Geometry check sheet. Reference: the model listing, model coordinates, mm. Face numbers are marked on the shaded views. A direction names the side the tool comes from. Coordinates: 2 decimals unless noted, no trailing zeros. Loops run counter-clockwise (first coordinate to the right, second up) from the corner with the lowest first, then second, coordinate; pieces in that order, holes last.
from build123d import *

# Parameters (mm, degrees)
SKETCH2_W           = 112.2
SKETCH2_H           = 87.2
SKETCH2_R           = 3
SKETCH2_W_2         = 71
SKETCH2_H_2         = 24
BOSS_EXTRUDE2_DEPTH = 60
SKETCH6_W           = 105
SKETCH6_H           = 80
CUT_EXTRUDE4_DEPTH  = 57.6
FILLET2_R           = 7
CUT_EXTRUDE5_REACH  = 89.2
SKETCH7_R           = 3
CUT_EXTRUDE6_REACH  = 114.2
SKETCH8_W           = 19.4
SKETCH8_H           = 6.4


with BuildPart() as part:
    # Sketch2 → Boss-Extrude2 (new body)
    with BuildSketch(Plane.XY):
        with Locations((3.248565438, 6.783112604)):
            Rectangle(SKETCH2_W, SKETCH2_H)
        with Locations((43.748565438, -12.816887396)):
            Circle(SKETCH2_R, mode=Mode.SUBTRACT)
        with Locations((-3.751434562, 8.383112604)):
            Rectangle(SKETCH2_W_2, SKETCH2_H_2, mode=Mode.SUBTRACT)
    extrude(amount=BOSS_EXTRUDE2_DEPTH)

    # Sketch6 → Cut-Extrude4 (cut)
    with BuildSketch(Plane(origin=(0, 0, 0), x_dir=(-1, 0, 0), z_dir=(0, 0, -1))):
        with Locations((-3.248565438, 6.783112604)):
            Rectangle(SKETCH6_W, SKETCH6_H)
    extrude(amount=-CUT_EXTRUDE4_DEPTH, mode=Mode.SUBTRACT)

    # Fillet2
    fillet2_edges = [part.edges().sort_by_distance(p)[0] for p in [
        (-52.851434562, 50.383112604, 30),
        (59.348565438, 50.383112604, 30),
        (59.348565438, -36.816887396, 30),
        (-52.851434562, -36.816887396, 30),
    ]]
    fillet(fillet2_edges, radius=FILLET2_R)

    # Sketch7 → Cut-Extrude5 (cut, up to next)
    with BuildSketch(Plane(origin=(0, 50.383112604, 0), x_dir=(1, 0, 0), z_dir=(0, 1, 0)), mode=Mode.PRIVATE) as cut_extrude5_sk1:
        with Locations((3.248565438, -30)):
            Circle(SKETCH7_R)
    cut_extrude5_tool1 = extrude(cut_extrude5_sk1.sketch, amount=-CUT_EXTRUDE5_REACH, mode=Mode.PRIVATE) & part.part
    add(cut_extrude5_tool1.solids().sort_by_distance((3.248565, 50.383113, 30))[0], mode=Mode.SUBTRACT)

    # Sketch8 → Cut-Extrude6 (cut, up to next)
    with BuildSketch(Plane.ZY.offset(52.851434562), mode=Mode.PRIVATE) as cut_extrude6_sk1:
        with Locations((13.1, -23.624199851)):
            Rectangle(SKETCH8_W, SKETCH8_H)
    cut_extrude6_tool1 = extrude(cut_extrude6_sk1.sketch, amount=-CUT_EXTRUDE6_REACH, mode=Mode.PRIVATE) & part.part
    add(cut_extrude6_tool1.solids().sort_by_distance((-52.851435, -23.6242, 13.1))[0], mode=Mode.SUBTRACT)


solid = part.part
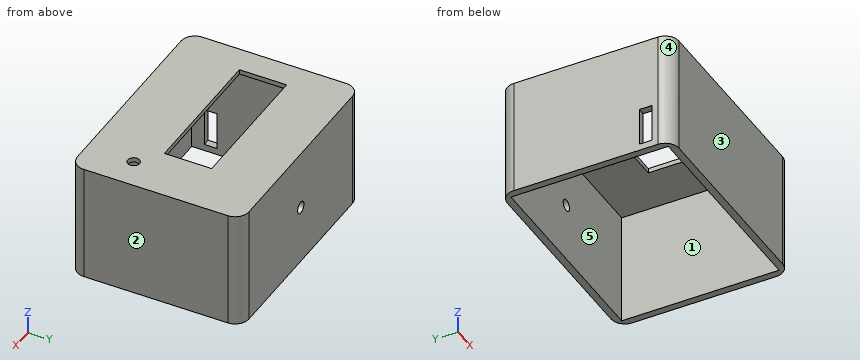
(1) Sectioned sample at A-A on y = 14. Record the cut outline in (x, z), and give its area (3 significant figures).
Findings:
outline: (-52.85, 0) - (-49.25, 0) - (-49.25, 57.6) - (-39.25, 57.6) - (-39.25, 60) - (-52.85, 60) - close; (31.75, 57.6) - (55.75, 57.6) - (55.75, 0) - (59.35, 0) - (59.35, 60) - (31.75, 60) - close
area: 514 mm2
(2) Sectioned sample at C-C on z = 44. Record the cut outline in (x, y), and give its area (3 significant figures).
Findings:
outline: (-52.85, -29.82) arc R7 ccw to (-45.85, -36.82) - (52.35, -36.82) arc R7 ccw to (59.35, -29.82) - (59.35, 43.38) arc R7 ccw to (52.35, 50.38) - (-45.85, 50.38) arc R7 ccw to (-52.85, 43.38) - close; hole (-49.25, -33.22) - (55.75, -33.22) - (55.75, 46.78) - (-49.25, 46.78) - close
area: 1,340 mm2
(3) Draft check along Y on the marked faces 1, 2 and 3. Enter one of: +Y half, -Y half, draft (parallel to the pull), parting line (faces both ways), or undercut.
Findings:
face 1: undercut
face 2: draft
face 3: -Y half
(4) Sectioned sample at D-D on z = 30. Record the cut outline in (x, y).
Findings:
outline: (-52.85, -29.82) arc R7 ccw to (-45.85, -36.82) - (52.35, -36.82) arc R7 ccw to (59.35, -29.82) - (59.35, 43.38) arc R7 ccw to (52.35, 50.38) - (6.25, 50.38) - (6.25, 46.78) - (55.75, 46.78) - (55.75, -33.22) - (-49.25, -33.22) - (-49.25, 46.78) - (0.25, 46.78) - (0.25, 50.38) - (-45.85, 50.38) arc R7 ccw to (-52.85, 43.38) - close
(5) Access from +Z, -Z, +X, -X, +Y, -Y to the whole of each face (thin tool, end or side, straight path). Record for the marked faces 4 and 5.
Findings:
face 4: +Z, -Z, -X, -Y
face 5: -Z
(6) Scan lines: L1, parallel to Y at x = 33, z = 12.5; L2, parallel to X at y = 44, z = 21; L3, parallel to X at y = 29.5, z = 3. Record each from-to range of solid material in increasing order.
Findings:
L1: y = -36.82 to -33.22, 46.78 to 50.38
L2: x = -52.82 to -49.25, 55.75 to 59.32
L3: x = -52.85 to -49.25, 55.75 to 59.35
(7) Sectioned sample at B-B on x = -28. Record the cut outline in (y, z), and give its area (3 significant figures).
Findings:
outline: (-36.82, 0) - (-33.22, 0) - (-33.22, 57.6) - (-3.62, 57.6) - (-3.62, 60) - (-36.82, 60) - close; (20.38, 57.6) - (46.78, 57.6) - (46.78, 0) - (50.38, 0) - (50.38, 60) - (20.38, 60) - close
area: 566 mm2
(8) Gauge pin test, flat ends, axial feed: pin 1 Ø8 at (x, y) = (-10.5, 15.5) entering from +Z; pin 2 Ø4 at (x, z) = (-50.5, 16) entering from +Y; pin 3 Ø3 at (x, z) = (-51, 9.5) entering from -Y; pin 4 Ø9.5 at (x, y) = (43.75, -12.82) entering from -Z. Record the tip position at first contact, or that the pin passes through.
Findings:
pin 1: passes through
pin 2: stops at y = 49.86
pin 3: stops at y = -35.79
pin 4: stops at z = 57.6
